Build history of the part. All positions in model axes, mm. A direction names the side the tool comes from. Coordinates: 2 decimals unless noted, no trailing zeros. Order: outer loops, then holes, each group sorted by start corner. A loop starts at its lowest first (then second) coordinate and runs counter-clockwise, first axis right, second up. Notation, with made-up numbers: (33.5, 38.25) - (79.5, 38.25) arc R12 ccw to (79.5, 50.25) - close; hole circle Ø10 at (41, 21.25). An arc over 180 degrees is marked (long way). Answer as CSV lines item,"result". Start each with the question number.
Autodesk Inventor part; units mm, degrees
ref_plane "Work Plane1" through (0, -18.5, 0) normal (0, 1, 0) x (-1, 0, 0)
ref_plane "YZ Plane" through (0, 0, 0) normal (1, 0, 0) x (0, 1, 0)
ref_plane "XY Plane" through (0, 0, 0) normal (0, 0, 1) x (1, 0, 0)
sketch "Sketch1" plane through (0, 0, 0) normal (0, 1, 0) x (-1, 0, 0)
  circle A0 centre (0, 0) radius 2.5
  circle A1 centre (0, 0) radius 2
  dimension "d0" = 5
  dimension "d1" = 4
sketch "Sketch2" plane through (0, 0, 0) normal (0, 0, 1) x (1, 0, 0)
  line L0 (0, 0) -> (0, 0)
  line L1 (7, -7) -> (25, -7)
  line L2 (32, 0) -> (32, 0)
  arc A0 (0, 0) -> (7, -7) centre (7, 0) ccw
  arc A1 (25, -7) -> (32, 0) centre (25, 0) ccw
  point P0 (0, -7)
  point P1 (32, -7)
  dimension "d3" = 32
  dimension "d4" = 7
  dimension "d5" = 7
sweep "Sweep1" add profiles "Sketch1" path "Sketch2"
ref_plane "Work Plane1" through (0, -18.5, 0) normal (0, 1, 0) x (-1, 0, 0)
sketch "Sketch3" plane through (0, -18.5, 0) normal (0, 1, 0) x (-1, 0, 0)
  circle A0 centre (-16, 0) radius 2.5
  circle A1 centre (0, 0) radius 2.5
  circle A2 centre (-16, 0) radius 2
  dimension "d9" = 5
  dimension "d10" = 16
  dimension "d11" = 4
extrude "Extrusion1" add sketch "Sketch3" along normal up to surface contours A0
properties part number "25"
(1) Which spindle directions (+Z, -Z, +X, -X, +Y, -Y) get a long thin tool onto all of the face, cutting with end or side? Do faces 1 (the cylindrical face through (16, -14, -2)), 2 (the flat face through (33, 0, -2)). Say none if no direction does.
(2) Probe L1, parallel to Z at x = 16, y = -14.5; L2, parallel to Y at x = 13, z = -0.1; L3, parallel to X at y = -15.25, z = 0. List the from-to ranges inside material, lowest first. Write a range as [from, to].
(3) Band-saw the part on C-C on y = -12. List the corners of the cut face in (x, z).
(4) Drop flat-ended pins along their axis: pin 1 Ø2.5 at (x, z) = (16, 0) entering from -Y; pin 2 Ø1 at (y, z) = (-7.5, 0) entering from -X; pin 3 Ø4 at (x, y) = (11, -14) entering from -Z. Give the stop position or say it passes through.
(5) Band-saw the part on A-A on x = 16. List the corners of the cut face in (y, z), plus the area to 3 significant figures.
(6) Band-saw the part on B-B on z = -0.4. List the corners of the cut face in (x, y), plus the area to 3 significant figures.
(7) Band-saw the part on D-D on z = 1.35. List the corners of the cut face in (x, y), plus the area to 3 significant figures.
(8) Pull direction Z, two halves, no side cores. Call faces 3 (the cylindrical face through (16, -5, 0)), 4 (the cylindrical face through (16.1, -4.5, -0.1)), 5 (the flat face through (17, -18.5, 2)), 6 (the cylindrical face through (16, -9.5, 0)): +Z half, -Z half, draft (parallel to the pull), parting line (faces both ways), or undercut.
Filled in:
1,face 1,"-Y"
1,face 2,"+Z, -Z, +X, -X, +Y"
2,L1,"z = [-2.5, -2], [2, 2.5]"
2,L2,"y = [-9.5, -9], [-5, -4.5]"
2,L3,"x = [13.5, 14], [18, 18.5]"
3,outline,"circle Ø5 at (16, 0); hole circle Ø4 at (16, 0)"
4,pin 1,"stops at y = -9.5"
4,pin 2,"stops at x = 0.58"
4,pin 3,"passes through"
5,outline,"(-18.5, -2.5) - (-7, -2.5) arc R2.5 ccw to (-7, 2.5) - (-18.5, 2.5) - (-18.5, 2) - (-8.5, 2) arc R2.5 ccw to (-8.5, -2) - (-18.5, -2) - close; hole circle Ø4 at (-7, 0)"
5,area,"17.5 mm^2"
6,outline,"(-2.47, 0) arc R9.47 ccw to (7, -9.47) - (13.53, -9.47) - (13.53, -18.5) - (14.04, -18.5) - (14.04, -9.47) - (17.96, -9.47) - (17.96, -18.5) - (18.47, -18.5) - (18.47, -9.47) - (25, -9.47) arc R9.47 ccw to (34.47, 0) - (33.96, 0) arc R8.96 cw to (25, -8.96) - (7, -8.96) arc R8.96 cw to (-1.96, 0) - close; (1.96, 0) arc R5.04 ccw to (7, -5.04) - (25, -5.04) arc R5.04 ccw to (30.04, 0) - (29.53, 0) arc R4.53 cw to (25, -4.53) - (7, -4.53) arc R4.53 cw to (2.47, 0) - close"
6,area,"49.8 mm^2"
7,outline,"(-2.1, 0) arc R9.1 ccw to (7, -9.1) - (13.9, -9.1) - (13.9, -18.5) - (14.52, -18.5) - (14.52, -9.1) - (17.48, -9.1) - (17.48, -18.5) - (18.1, -18.5) - (18.1, -9.1) - (25, -9.1) arc R9.1 ccw to (34.1, 0) - (33.48, 0) arc R8.48 cw to (25, -8.48) - (7, -8.48) arc R8.48 cw to (-1.48, 0) - close; (1.48, 0) arc R5.52 ccw to (7, -5.52) - (25, -5.52) arc R5.52 ccw to (30.52, 0) - (29.9, 0) arc R4.9 cw to (25, -4.9) - (7, -4.9) arc R4.9 cw to (2.1, 0) - close"
7,area,"62.1 mm^2"
8,face 3,"undercut"
8,face 4,"parting line"
8,face 5,"draft"
8,face 6,"undercut"
